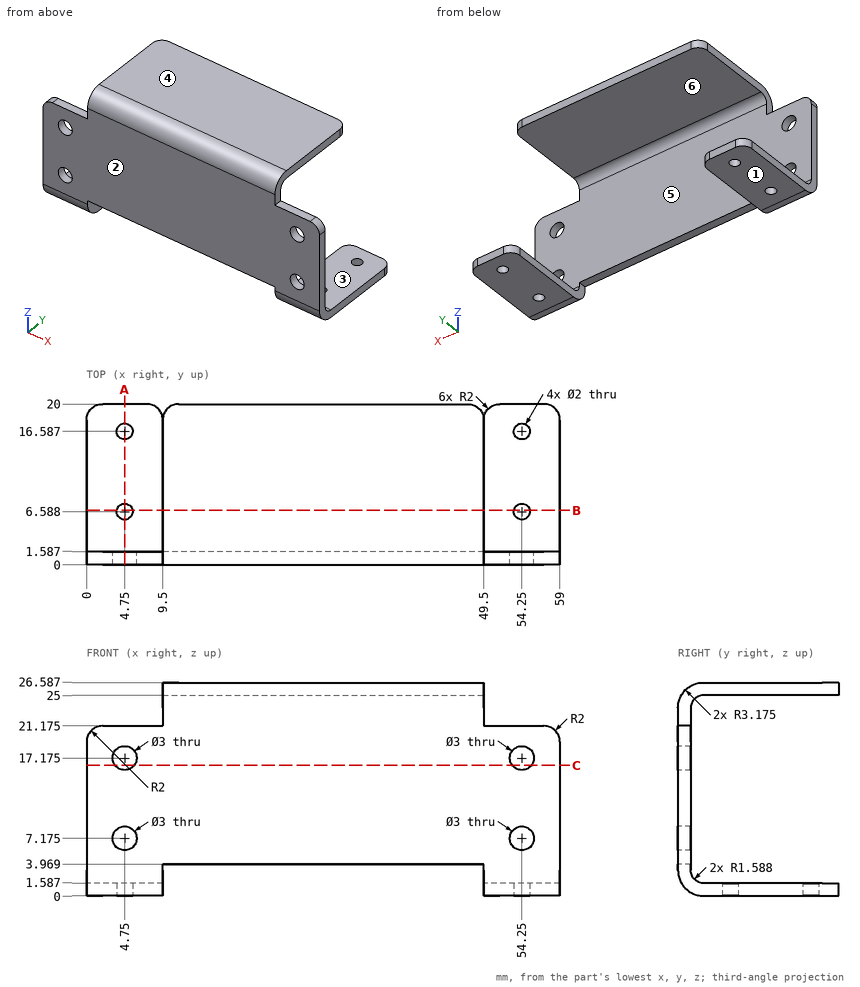
Part print with two shaded views. Sizes in mm from the minimum x, y, z corner. A direction names the side the tool comes from. Give positions to 0.01 mm unless a question says otherwise; leave off trailing zeros. Loops run counter-clockwise (first coordinate to the right, second up) from the corner with the lowest first, then second, coordinate; pieces in that order, holes last. Notation, with made-up numbers: (10, 53.5) - (33, 53.5) arc R16 cw to (33, 71.5) - close; hole circle Ø4 at (70.5, 27.5). An arc over 180 degrees is marked (long way). Put each result on its own line as item: value.
Q1. Slice it at A-A (x = 4.75). Give the number of separate pieces and of enclosed holes in the cut face.
Filled in:
separate pieces: 5
enclosed holes: 0
Q2. Slice it at B-B (y = 6.75). Give the cut face in (x, z).
Filled in:
outline: (0, 0) - (3.76, 0) - (3.76, 1.59) - (0, 1.59) - close; (5.74, 0) - (9.5, 0) - (9.5, 1.59) - (5.74, 1.59) - close; (9.5, 25) - (49.5, 25) - (49.5, 26.59) - (9.5, 26.59) - close; (49.5, 0) - (53.26, 0) - (53.26, 1.59) - (49.5, 1.59) - close; (55.24, 0) - (59, 0) - (59, 1.59) - (55.24, 1.59) - close
Q3. Tool access for the marked faces 4, 5 and 6: list every direction of +Z, -Z, +X, -X, +Y, -Y with a clear straight run to the whole face (end or side of a thin tool).
Filled in:
face 4: +Z, +X, -X, +Y, -Y
face 5: +X, -X, +Y
face 6: -Z, +X, -X, +Y
Q4. Mould opens along Z. For the marked faces 1, 2 and 3 say: pulls with the +Z half, pulls with the -Z half, needs draft (parallel to the pull), parting line crosses it, or undercut.
Filled in:
face 1: pulls with the -Z half
face 2: needs draft
face 3: pulls with the +Z half
Q5. Slice it at C-C (z = 16.25). Give the cut face in (x, y).
Filled in:
outline: (0, 0) - (3.57, 0) - (3.57, 1.59) - (0, 1.59) - close; (5.93, 0) - (53.07, 0) - (53.07, 1.59) - (5.93, 1.59) - close; (55.43, 0) - (59, 0) - (59, 1.59) - (55.43, 1.59) - close
Q6. Probe line 1 along Z through (x, y) = (54.25, 0.9) (1 decimal); line 2 along Z through (x, y) = (54.25, 1) (1 decimal); line 3 along Y through (x, z) = (46, 7.5). List the from-to ranges inside material, lowest first.
Filled in:
line 1: z = 1 to 5.7, 8.7 to 15.7, 18.7 to 21.2
line 2: z = 0.9 to 5.7, 8.7 to 15.7, 18.7 to 21.2
line 3: y = 0 to 1.59
Q7. Flat gauge pins, fed straight in: pin 1 (5 mm diameter, centred on x = 56.5, y = 10, fed in from +Z); pin 2 (5 mm diameter, centred on x = 32, y = 8.5, fed in from -Z); pin 3 (4.5 mm diameter, centred on y = 10.5, z = 23.5, fed in from +X). Where does each tip first touch, or does it go through?
Filled in:
pin 1: stops at z = 1.59
pin 2: stops at z = 25
pin 3: stops at x = 49.5
